from build123d import *

# Parameters (mm, degrees)
ESQUISSE1_W      = 150
ESQUISSE1_H      = 2
ESQUISSE2_R      = 5
EXTRUSION1_DEPTH = 15


with BuildPart() as part:
    # Esquisse1 → Révolution1 (revolve)
    with BuildSketch(Plane.XY, mode=Mode.PRIVATE) as r_volution1_sk:
        with Locations((75, 1)):
            Rectangle(ESQUISSE1_W, ESQUISSE1_H)
    revolve(r_volution1_sk.sketch.rotate(Axis((0, 0, 0), (1, 0, 0)), 90), axis=Axis((0, 0, 0), (1, 0, 0)))  # turned: the seam where the file's is

    # Esquisse2 → Extrusion1 (add, symmetric)
    with BuildSketch(Plane.XY):
        with Locations((90, 0)):
            Circle(ESQUISSE2_R)
        with Locations((25, 0)):
            Circle(ESQUISSE2_R)
    extrude(amount=EXTRUSION1_DEPTH, both=True)


solid = part.part
The model under review builds one solid part; all positions refer to its coordinate system, in mm. A direction names the side the tool comes from. Give positions to 0.01 mm unless a question says otherwise; leave off trailing zeros. Loops run counter-clockwise (first coordinate to the right, second up) from the corner with the lowest first, then second, coordinate; pieces in that order, holes last. Notation, with made-up numbers: (-5, 75) -> (14, 75) arc R18 cw to (14, 86) -> close; hole circle Ø3 at (-27.5, 13). An arc over 180 degrees is marked (long way). Write each question's results on one line, items separated by ' | '.
1) Take a section at B-B, the plane z = -4. Give the boundary of the cut face in (x, y).
Conclusion:
outline: circle Ø10 at (25, 0); circle Ø10 at (90, 0)
2) Take a section at A-A, the plane y = 0. Give the boundary of the cut face in (x, z), plus the area to 3 significant figures.
Conclusion:
outline: (0, -2) -> (20, -2) -> (20, -15) -> (30, -15) -> (30, -2) -> (85, -2) -> (85, -15) -> (95, -15) -> (95, -2) -> (150, -2) -> (150, 2) -> (95, 2) -> (95, 15) -> (85, 15) -> (85, 2) -> (30, 2) -> (30, 15) -> (20, 15) -> (20, 2) -> (0, 2) -> close | area: 1,120 mm^2
3) Draft analysis for pull direction X (two halves, no side actions). For faces 1 (the face through (90, 0, -15)), 2 (the face through (150, 0, 0)), 3 (the face through (58, 2, 0)), 4 (the face through (0, 0, 0)), state which applies: pulls with the +X half, pulls with the -X half, needs draft (parallel to the pull), parting line crosses it, or undercut.
Conclusion:
face 1: needs draft | face 2: pulls with the +X half | face 3: undercut | face 4: pulls with the -X half
4) Take a section at C-C, the plane x = 45.5. Give the boundary of the cut face in (y, z).
Conclusion:
outline: circle Ø4 at (0, 0)
5) For line 1 along X through (y, z) = (2, 2.5); line 2 along Z through (x, y) = (68, 0.25); line 3 along X through (y, z) = (-1.5, 8), list the stretches that pass through material, from the lowest coordinate up. Write a range as from..to.
Conclusion:
line 1: x = 20.42..29.58, 85.42..94.58 | line 2: z = -1.98..1.98 | line 3: x = 20.23..29.77, 85.23..94.77
6) Insertion check: pin 1 Ø8 at (x, z) = (85.5, 8) entering from +Y; pin 2 Ø10 at (x, z) = (83.5, -10) entering from +Y. Each pin has a flat end and moves straight along its axis. Give the tip position at first contact, or say it passes through.
Conclusion:
pin 1: stops at y = 4.97 | pin 2: stops at y = 4.77
7) Tool access review of faces 5 (the face through (10, 2, 0)), 6 (the face through (25, 0, 15)), 7 (the face through (123, 2, 0)), 8 (the face through (25, 0, -15)), 9 (the face through (21, -3, 0)): name each direction out of +Z, -Z, +X, -X, +Y, -Y from which nothing blocks a thin tool from reaching the whole face with its end or side.
Conclusion:
face 5: -X | face 6: +Z, +X, -X, +Y, -Y | face 7: +X | face 8: -Z, +X, -X, +Y, -Y | face 9: none
